The listing builds one solid part. Answer for the finished solid, in the listing's coordinates (mm). Face numbers are marked on the shaded views. A direction names the side the tool comes from. Give positions to 0.01 mm unless a question says otherwise; leave off trailing zeros. Loops run counter-clockwise (first coordinate to the right, second up) from the corner with the lowest first, then second, coordinate; pieces in that order, holes last. Notation, with made-up numbers: (21, 39.25) - (33, 39.25) arc R27 ccw to (33, 78.25) - close; hole circle Ø10 at (-35.5, 46.5). An arc over 180 degrees is marked (long way). Write each question's results on one line, items separated by ' | '.
from build123d import *

# Parameters (mm, degrees)
F2_R          = 40.1855244707
F3_DEPTH      = 25.4
F4_R          = 6.35
F5_DEPTH      = 48.26
F5_DEPTH_BACK = 48.26
F6_DEPTH      = 12.7
F6_DEPTH_BACK = 12.7


# Not quite as in the source:
# - ends of sketch curves that miss each other by under 0.0002 mm in the source are joined


with BuildPart() as f1:
    # F0 (on Front) → F1 (revolve)
    with BuildSketch(Plane.XZ):
        Polygon((0, 50.8), (0, 0), (127, 0), (127, 50.8), (43.18, 50.8), (43.18, 48.26), (40.64, 48.26), (40.64, 50.8), (27.94, 50.8), (27.94, 48.26), (25.4, 48.26), (25.4, 50.8), align=None)
    revolve(axis=Axis((-13.3472196758, 0, 0), (1, 0, 0)))

    # F2 (on face) → F3 (cut)
    with BuildSketch(Plane.YZ.offset(127)):
        Circle(F2_R)
    extrude(amount=-F3_DEPTH, mode=Mode.SUBTRACT)

    # F4 (on Front) → F5 (join, two sides)
    with BuildSketch(Plane.XZ) as f5_sk:
        with BuildLine():
            Line((101.6, -12.7), (114.3, -12.7))
            ThreePointArc((114.3, -12.7), (127.0000011214, 0), (114.3, 12.7000011214))
            Line((114.3, 12.7000011214), (101.6, 12.7))
            Line((101.6, 12.7), (101.6, -12.7))
        make_face()
        with Locations((114.3, 0)):
            Circle(F4_R, mode=Mode.SUBTRACT)
    extrude(amount=F5_DEPTH)
    extrude(f5_sk.sketch, amount=-F5_DEPTH_BACK)

    # F4 (on Front) → F6 (cut, two sides)
    with BuildSketch(Plane.XZ) as f6_sk:
        with BuildLine():
            Line((101.6, -12.7), (114.3, -12.7))
            ThreePointArc((114.3, -12.7), (127.0000011214, 0), (114.3, 12.7000011214))
            Line((114.3, 12.7000011214), (101.6, 12.7))
            Line((101.6, 12.7), (101.6, -12.7))
        make_face()
        with Locations((114.3, 0)):
            Circle(F4_R, mode=Mode.SUBTRACT)
    extrude(amount=-F6_DEPTH, mode=Mode.SUBTRACT)
    extrude(f6_sk.sketch, amount=F6_DEPTH_BACK, mode=Mode.SUBTRACT)

    # F7 (on Front) → F8 (revolve, cut)
    with BuildSketch(Plane.XZ):
        Polygon((0, 50.5328811705), (0, 0), (9.8897889256, 0), align=None)
    revolve(axis=Axis((4.9448944628, 0, 0), (-1, 0, 0)), mode=Mode.SUBTRACT)


solid = f1.part
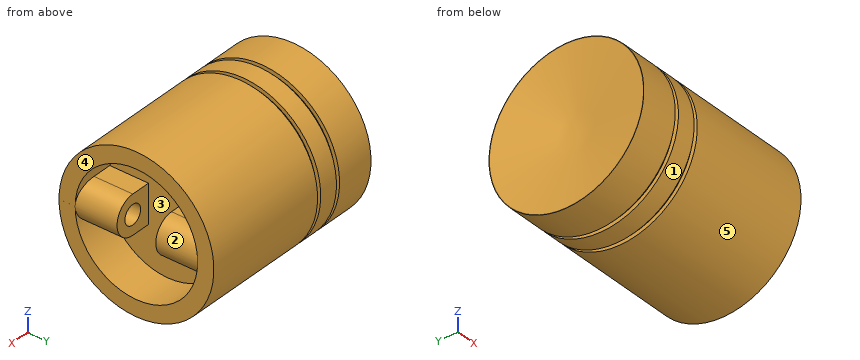
Item 1: A cutting plane is placed at B-B, the plane x = 87. Determine the outline of the cut face in (y, z).
Values found:
outline: circle Ø101.6 at (0, 0)
Item 2: For the marked faces 1 and 2, determine the directions among +Z, -Z, +X, -X, +Y, -Y from which every point of the face is accessible in a straight line to the end or side of a thin tool.
Values found:
face 1: +X, -X | face 2: +X
Item 3: Find the intervals of material crossed by line 1 along Z through (x, y) = (114.3, 24.5); line 2 along X through (y, z) = (-18, -46); line 3 along X through (y, z) = (-18, 0), in increasing order. Write a range as [from, to].
Values found:
line 1: z = [-44.5, -31.85], [-12.7, -6.35], [6.35, 12.7], [31.85, 44.5] | line 2: x = [0.22, 25.4], [27.94, 40.64], [43.18, 127] | line 3: x = [6.37, 107.95], [120.65, 127]
Item 4: A cutting plane is placed at A-A, the plane x = 111. Determine the outline of the cut face in (y, z).
Values found:
outline: circle Ø101.6 at (0, 0); hole (-39.82, -5.43) - (-12.7, -5.43) - (-12.7, -12.7) - (-38.13, -12.7) arc R40.19 ccw to (38.13, -12.7) - (12.7, -12.7) - (12.7, -5.43) - (39.82, -5.43) arc R40.19 ccw to (39.82, 5.43) - (12.7, 5.43) - (12.7, 12.7) - (38.13, 12.7) arc R40.19 ccw to (-38.13, 12.7) - (-12.7, 12.7) - (-12.7, 5.43) - (-39.82, 5.43) arc R40.19 ccw to start
Item 5: Flat-ended cylindrical pins translate along their axes: P1, Ø12.5, axis at x = 113.5, z = 3, coming from the +Y side; P2, Ø7.5, axis at x = 117.5, z = 5.5, coming from the -Y side; P3, Ø8, axis at x = 25.5, z = 10.5, coming from the +Y side. Find the tip coordinate at first contact, or state that the pin passes through.
Values found:
P1: stops at y = 50.8 | P2: stops at y = -50.77 | P3: stops at y = 50.38
Item 6: For a pull along Z with two mould halves and no side action, classify the marked faces 3, 4 and 5 as released by +Z, released by -Z, zero draft, split by the parting line, or undercut.
Values found:
face 3: undercut | face 4: zero draft | face 5: split by the parting line
